Could you check a few things on this model? Use its own coordinates, in mm. A direction names the side the tool comes from. Coordinates: 2 decimals unless noted, no trailing zeros. Order: outer loops, then holes, each group sorted by start corner. A loop starts at its lowest first (then second) coordinate and runs counter-clockwise, first axis right, second up. Notation, with made-up numbers: (-8.5, -38.5) -> (0.5, -38.5) arc R22 cw to (0.5, -2.5) -> close; hole circle Ø4 at (30.25, -9.75). An arc over 180 degrees is marked (long way). Use a Markdown table: item, result. Add a question column.
1) If we section it at C-C (y = 70): Write out the boundary of the cut face in (x, z), plus the area to 3 significant figures.
2) If I drill on L1, parallel to X at y = 60, z = -5; L2, parallel to Z at x = 5, y = 53; L3, parallel to Y at x = 55, z = -41, over which ranges is the centre line in solid material (lowest first)? Write a range as [from, to].
3) If we section it at A-A (x = 5): Write out the boundary of the cut face in (y, z), plus the area to 3 significant figures.
4) Which directions (+Z, -Z, +X, -X, +Y, -Y) give clear straight access to the entire face, cutting with the end or side of a thin tool? Please do faces 4 (the flat face through (83, 74.496, -43)), 5 (the flat face through (83, 55.446, -43)), 6 (the flat face through (76.284, 13, -43)).
5) If we section it at B-B (z = -20.75): Write out the boundary of the cut face in (x, y) (3 decimals).
6) If we section it at D-D (x = 66): Write out the boundary of the cut face in (y, z), plus the area to 3 significant figures.
7) Will these pins go through, and if not, where does the flat tip stop? pin 1 Ø0.8 at (y, z) = (66.5, -42.5) entering from -X; pin 2 Ø12.5 at (x, z) = (64.5, -10.5) entering from -Y; pin 3 Ø3 at (y, z) = (15.5, -42.5) entering from +X.
8) Thinking about a two-plate mould opening in X: for faces 1 (the flat face through (83, 22.496, -43)), 2 (the flat face through (6.284, 13, -43)), 3 (the flat face through (18.984, 13, -43)), which applies, +X half, -X half, draft (parallel to the pull), parting line (faces both ways), or undercut?
```python
from build123d import *

# Parameters (mm, degrees)
BOSS_EXTRUDE1_DEPTH         = 79
SKETCH2_W                   = 12.7
SKETCH2_H                   = 19.05
BOSS_EXTRUDE2_DEPTH         = 2.7
LPATTERN1_COUNT             = 2
LPATTERN1_PITCH             = 70
LPATTERN1_COUNT_DIR2        = 2
LPATTERN1_PITCH_DIR2        = 52
SKETCH3_R                   = 15
BOSS_EXTRUDE3_DEPTH         = 15
SKETCH4_R                   = 6.35
BOSS_EXTRUDE4_DEPTH         = 15
CUT_EXTRUDE1_DEPTH          = 131.826000856
TAP_DRILL_FOR_M3X0_5_TAP1_D = 2.5


with BuildPart() as part:
    # Sketch1 → Boss-Extrude1 (new body)
    with BuildSketch(Plane(origin=(0, 0, 0), x_dir=(1, 0, 0), z_dir=(0, 1, 0))):
        Polygon((0, 39.5), (2, 41.5), (92.45, 41.5), (94.45, 39.5), (94.45, 2), (92.45, 0), (2, 0), (0, 2), align=None)
    extrude(amount=BOSS_EXTRUDE1_DEPTH)

    # Sketch2 → Boss-Extrude2 (add)
    with BuildSketch(Plane(origin=(0, 0, -41.5), x_dir=(-1, 0, 0), z_dir=(0, 0, -1))):
        with Locations((-12.634045562, 12.971461945)):
            Rectangle(SKETCH2_W, SKETCH2_H)
    boss_extrude2 = extrude(amount=BOSS_EXTRUDE2_DEPTH)

    # LPattern1: Boss-Extrude2 2 × 2
    with Locations(*[(i * LPATTERN1_PITCH, j * LPATTERN1_PITCH_DIR2, 0) for i in range(LPATTERN1_COUNT) for j in range(LPATTERN1_COUNT_DIR2) if (i, j) != (0, 0)]):
        add(boss_extrude2)

    # Sketch3 → Boss-Extrude3 (add)
    with BuildSketch(Plane.XZ):
        with Locations(Location((47.225, -20.75, 0), (0, 0, 270))):
            Circle(SKETCH3_R)
    extrude(amount=BOSS_EXTRUDE3_DEPTH)

    # Sketch4 → Boss-Extrude4 (add)
    with BuildSketch(Plane.XZ.offset(15)):
        with Locations(Location((47.225, -20.75, 0), (0, 0, 270))):
            Circle(SKETCH4_R)
    extrude(amount=BOSS_EXTRUDE4_DEPTH)

    # Sketch5 → Cut-Extrude1 (cut, through all)
    with BuildSketch(Plane.XY):
        with BuildLine():
            Line((70.975, 7), (23.475, 7))
            ThreePointArc((23.475, 7), (22.414339828, 7.439339828), (21.975, 8.5))
            Line((21.975, 8.5), (21.975, 9.1))
            ThreePointArc((21.975, 9.1), (22.414339828, 10.160660172), (23.475, 10.6))
            Line((23.475, 10.6), (70.975, 10.6))
            ThreePointArc((70.975, 10.6), (72.035660172, 10.160660172), (72.475, 9.1))
            Line((72.475, 9.1), (72.475, 8.5))
            ThreePointArc((72.475, 8.5), (72.035660172, 7.439339828), (70.975, 7))
        make_face()
    extrude(amount=-CUT_EXTRUDE1_DEPTH, mode=Mode.SUBTRACT)

    # Tap Drill for M3x0.5 Tap1 (through all)
    with Locations(Plane(origin=(0, 0, 0), x_dir=(-1, 0, 0), z_dir=(0, -1, 0))):
        with Locations((-5, 5), (-5, 36.5), (-89.45, 36.5), (-89.45, 5)):
            Hole(TAP_DRILL_FOR_M3X0_5_TAP1_D / 2)


solid = part.part
```
Answer sheet:
| question | item | result |
|---|---|---|
| 1 | outline | (0, -39.5) -> (2, -41.5) -> (6.28, -41.5) -> (6.28, -44.2) -> (18.98, -44.2) -> (18.98, -41.5) -> (76.28, -41.5) -> (76.28, -44.2) -> (88.98, -44.2) -> (88.98, -41.5) -> (92.45, -41.5) -> (94.45, -39.5) -> (94.45, -2) -> (92.45, 0) -> (2, 0) -> (0, -2) -> close; hole circle Ø2.5 at (5, -36.5); hole circle Ø2.5 at (5, -5); hole circle Ø2.5 at (89.45, -36.5); hole circle Ø2.5 at (89.45, -5) |
| 1 | area | 3,960 mm2 |
| 2 | L1 | [0, 3.75], [6.25, 88.2], [90.7, 94.45] |
| 2 | L2 | [-41.5, -37.75], [-35.25, -6.25], [-3.75, 0] |
| 2 | L3 | [0, 7], [10.6, 79] |
| 3 | outline | (0, -41.5) -> (79, -41.5) -> (79, -37.75) -> (0, -37.75) -> close; (0, -35.25) -> (79, -35.25) -> (79, -6.25) -> (0, -6.25) -> close; (0, -3.75) -> (79, -3.75) -> (79, 0) -> (0, 0) -> close |
| 3 | area | 2,880 mm2 |
| 4 | face 4 | -Z, +X, -X, +Y |
| 4 | face 5 | -Z, +X, -X |
| 4 | face 6 | -Z, +Y, -Y |
| 5 | outline | (0, 0) -> (32.225, 0) -> (32.225, -15) -> (40.875, -15) -> (40.875, -30) -> (53.575, -30) -> (53.575, -15) -> (62.225, -15) -> (62.225, 0) -> (94.45, 0) -> (94.45, 79) -> (0, 79) -> close; hole (21.975, 8.5) arc R1.5 ccw to (23.475, 7) -> (70.975, 7) arc R1.5 ccw to (72.475, 8.5) -> (72.475, 9.1) arc R1.5 ccw to (70.975, 10.6) -> (23.475, 10.6) arc R1.5 ccw to (21.975, 9.1) -> close |
| 6 | outline | (0, -41.5) -> (7, -41.5) -> (7, 0) -> (0, 0) -> close; (10.6, -41.5) -> (79, -41.5) -> (79, 0) -> (10.6, 0) -> close |
| 6 | area | 3,130 mm2 |
| 7 | pin 1 | x = 6.28 |
| 7 | pin 2 | y = -15 |
| 7 | pin 3 | x = 92.95 |
| 8 | face 1 | draft |
| 8 | face 2 | -X half |
| 8 | face 3 | undercut |
